Verification items for the finished model (mm, model axes). Face numbers are marked on the shaded views. A direction names the side the tool comes from. Round coordinates to 2 decimals unless told otherwise and drop trailing zeros. Write each loop counter-clockwise with the first axis right and the second up, starting at its lowest first coordinate (ties: lowest second). Pieces come first, ordered by that corner, then holes. Notation, with made-up numbers: M 61.25,-7 L 68.25,-7 A33 ccw 68.25,32 Z; hole C 58.5,31 d3. An arc over 180 degrees is marked long. Write each question's results on one line, items separated by ' | '.
Autodesk Inventor part; units mm, degrees
ref_plane "YZ Plane" through (0, 0, 0) normal (1, 0, 0) x (0, 1, 0)
ref_plane "XZ Plane" through (0, 0, 0) normal (0, 1, 0) x (-1, 0, 0)
ref_plane "XY Plane" through (0, 0, 0) normal (0, 0, 1) x (1, 0, 0)
sketch "Boceto1" plane through (0, 0, 0) normal (0, 1, 0) x (-1, 0, 0)
  line L0 (-20, 20) -> (20, 20)
  line L1 (20, 20) -> (20, -20)
  line L2 (20, -20) -> (-20, -20)
  line L3 (-20, -20) -> (-20, 20)
  line L4 (-20, 20) -> (20, -20) construction
  line L5 (20, 20) -> (-20, -20) construction
  point P0 (0, 0)
  dimension "d0" = 40
  dimension "d1" = 40
extrude "Extrusión1" add sketch "Boceto1" along normal blind 6
sketch "Boceto2" plane through (0, 6, 0) normal (0, 1, 0) x (1, 0, 0)
  line L0 (15.5, -15.5) -> (-15.5, -15.5)
  line L1 (-15.5, -15.5) -> (-15.5, 15.5)
  line L2 (-15.5, 15.5) -> (15.5, 15.5)
  line L3 (15.5, 15.5) -> (15.5, -15.5)
  line L4 (15.5, -15.5) -> (-15.5, 15.5) construction
  line L5 (-15.5, -15.5) -> (15.5, 15.5) construction
  point P0 (0, 0)
  dimension "d4" = 31
  dimension "d5" = 31
hole "Agujero1" at (-15.5, 6, 15.5) at (-15.5, 6, -15.5) at (15.5, 6, -15.5) at (15.5, 6, 15.5) direction (0, -1, 0) diameter 3 depth 8 tip angle 118
sketch "Boceto3" plane through (0, 6, 0) normal (0, 1, 0) x (1, 0, 0)
  circle A0 centre (0, 0) radius 12.7
  dimension "d13" = 25.4
extrude "Extrusión2" add sketch "Boceto3" along normal blind 18
sketch "Boceto4" plane through (0, 24, 0) normal (0, 1, 0) x (1, 0, 0)
  point P0 (0, 0)
  point P1 (0, 0)
hole "Agujero2" at (0, 24, 0) direction (0, -1, 0) diameter 12 depth 8
properties part number "SoporteVarilla"
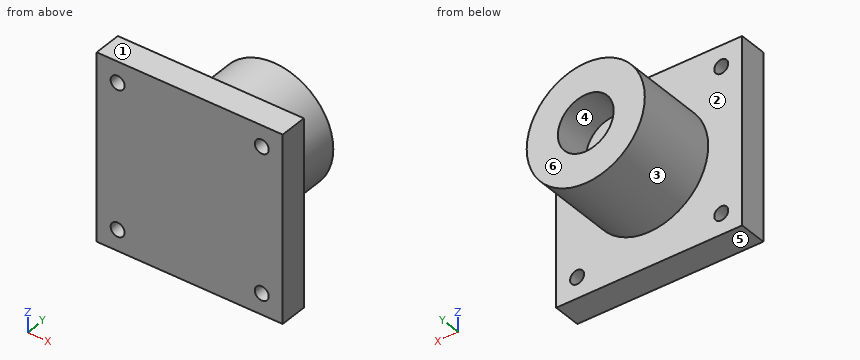
1) Sectioned sample at C-C, the plane z = 0. Record the cut outline in (x, y).
Calculated:
outline: M -20,0 L 20,0 L 20,6 L 12.7,6 L 12.7,24 L 6,24 L 6,16 L -6,16 L -6,24 L -12.7,24 L -12.7,6 L -20,6 Z
2) Depth check by flat-ended pin: P1, Ø5, axis at x = -7.5, y = 21.5, coming from the -Z side; P2, Ø10, axis at y = 15.5, z = -12.5, coming from the -X side; P3, Ø3, axis at x = 2, y = 18.5, coming from the +Z side. Enter the tip coordinate at first touch or a pass-through.
Calculated:
P1: stops at z = -11.67 | P2: stops at x = -10.25 | P3: stops at z = 12.69
3) Sectioned sample at A-A, the plane x = -15.5. Record the cut outline in (y, z), and give its area (3 significant figures).
Calculated:
outline: M 0,-20 L 6,-20 L 6,-17 L 0,-17 Z; M 0,-14 L 6,-14 L 6,14 L 0,14 Z; M 0,17 L 6,17 L 6,20 L 0,20 Z | area: 204 mm²
4) Access from +Z, -Z, +X, -X, +Y, -Y to the whole of each face (thin tool, end or side, straight path). Record for the marked faces 1 and 2.
Calculated:
face 1: +Z, +X, -X, +Y, -Y | face 2: +Y
5) Material ranges on line 1 (Z direction, x = -15.5, y = 4.75); line 2 (X direction, y = 21.75, z = 0), recorded low to high. Write a range as [from, to].
Calculated:
line 1: z = [-20, -17], [-14, 14], [17, 20] | line 2: x = [-12.7, -6], [6, 12.7]
6) Sectioned sample at D-D, the plane x = 0. Record the cut outline in (y, z).
Calculated:
outline: M 0,-20 L 6,-20 L 6,-12.7 L 24,-12.7 L 24,-6 L 16,-6 L 16,6 L 24,6 L 24,12.7 L 6,12.7 L 6,20 L 0,20 Z
7) Sectioned sample at B-B, the plane z = -15.5. Record the cut outline in (x, y), and give its area (3 significant figures).
Calculated:
outline: M -20,0 L -17,0 L -17,6 L -20,6 Z; M -14,0 L 14,0 L 14,6 L -14,6 Z; M 17,0 L 20,0 L 20,6 L 17,6 Z | area: 204 mm²
8) Draft check along Z on the marked faces 3, 4, 5 and 6. Enter one of: pulls with the +Z half, pulls with the -Z half, needs draft (parallel to the pull), parting line crosses it, or undercut.
Calculated:
face 3: parting line crosses it | face 4: undercut | face 5: pulls with the -Z half | face 6: needs draft
